Could you check a few things on this model? Use its own coordinates, in mm. Face numbers are marked on the shaded views. A direction names the side the tool comes from. Round coordinates to 2 decimals unless told otherwise and drop trailing zeros. Write each loop counter-clockwise with the first axis right and the second up, starting at its lowest first coordinate (ties: lowest second). Pieces come first, ordered by that corner, then holes. Notation, with made-up numbers: (22, 62.25) -> (35, 62.25) arc R17 cw to (35, 75.25) -> close; hole circle Ø3 at (-36, 65). An arc over 180 degrees is marked (long way). Answer as CSV lines item,"result". Start each with the question number.
Q1. Imagine slicing it at A-A on y = 5. Please give me the cut outline in (x, z).
Q2. Imagine slicing it at C-C on y = -3.5. Please give me the cut outline in (x, z) (3 decimals), and give its area (3 significant figures).
Q3. Will these pins go through, and if not, where does the flat tip stop? pin 1 Ø12 at (y, z) = (9, 8) entering from +X; pin 2 Ø4 at (y, z) = (42.5, 3) entering from +X; pin 3 Ø1.5 at (x, z) = (4, 13.5) entering from -Y; pin 4 Ø1.5 at (x, y) = (2.5, 5) entering from -Z.
Q4. If I drill on line 1 (Y direction, x = 11.7, z = 2.5) (3 decimals); line 2 (Z direction, x = 7.25, y = 1); line 3 (X direction, y = 34, z = -0.25), over which ranges is the centre line in solid material (lowest first)? Write a range as [from, to].
Q5. If we mould it in two halves opening along Z, with no side actions, what happens to the marked faces 6, 7, 8 and 9? For each: pulls with the +Z half, pulls with the -Z half, needs draft (parallel to the pull), parting line crosses it, or undercut.
Q6. Imagine slicing it at B-B on z = 7.5. Please give me the cut outline in (x, y).
Q7. Imagine slicing it at D-D on x = 14.25. Please give me the cut outline in (y, z).
Q8. For the marked faces 1, 2, 3, 4 and 5, which set-ups out of +Z, -Z, +X, -X, +Y, -Y let a thin tool reach every point of the face, with its end or its side?
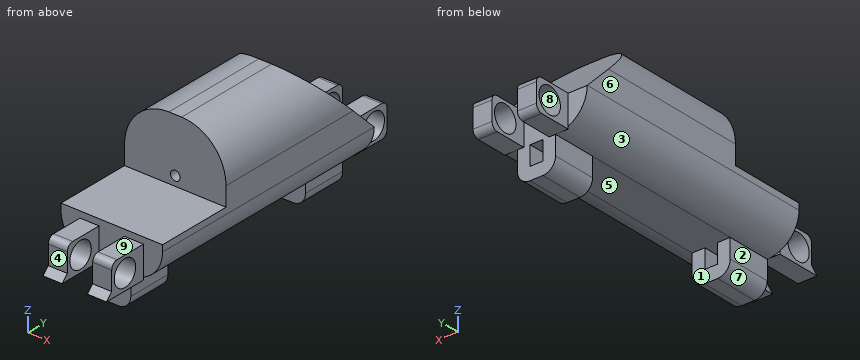
Autodesk Inventor part; units mm, degrees
ref_plane "YZ Plane" through (0, 0, 0) normal (1, 0, 0) x (0, 1, 0)
ref_plane "XZ Plane" through (0, 0, 0) normal (0, 1, 0) x (-1, 0, 0)
ref_plane "XY Plane" through (0, 0, 0) normal (0, 0, 1) x (1, 0, 0)
sketch "Sketch2" plane through (0, 0, 0) normal (0, 0, 1) x (1, 0, 0)
  line L0 (0, 0) -> (16, 0)
  line L1 (16, 0) -> (16, 40)
  line L2 (16, 40) -> (0, 40)
  line L3 (0, 40) -> (0, 0)
  dimension "d0" = 16
  dimension "d1" = 40
extrude "Extrusion1" add sketch "Sketch2" along normal blind 16
fillet "Fillet1" radius 7 2 edges at (16, 20, 16) (0, 20, 16)
fillet "Fillet2" radius 5 2 edges at (16, 20, 0) (0, 20, 0)
sketch "Sketch3" plane through (16, 0, 9) normal (1, 0, 0) x (0, 0, -1)
  line L0 (4, 0) -> (4, 40)
  line L1 (4, 40) -> (-7, 29)
  line L2 (-7, 0) -> (-7, 40)
  line L3 (4, 40) -> (19.5563, 40) construction
  line L4 (-7, 29) -> (-7, 40)
  line L5 (-7, 40) -> (4, 40)
  line L6 (1, 0) -> (12.3137, 0) construction
  line L7 (-7, 8) -> (-7, 0)
  line L8 (1, 0) -> (19.9296, 0) construction
  line L9 (-7, 17.1561) -> (-7, 8)
  point P0 (9, 0)
  dimension "d6" = 135
extrude "Extrusion2" cut sketch "Sketch3" against normal through all
sketch "Sketch4" plane through (5, 40, 0) normal (0, 1, 0) x (1, 0, 0)
  line L0 (1, -4.25) -> (5, -0.75) construction
  line L1 (-5, -5) -> (11, -5)
  line L2 (1, -5) -> (-2, -5)
  line L3 (-2, -5) -> (-2, 0)
  line L4 (-2, 0) -> (1, 0)
  line L5 (1, 0) -> (1, -5)
  line L6 (5, 0) -> (8, 0)
  line L7 (8, 0) -> (8, -5)
  line L8 (8, -5) -> (5, -5)
  line L9 (5, -5) -> (5, 0)
  point P0 (-5, 0)
  point P1 (-1.888, -0.75)
  point P2 (-1.888, -4.25)
  dimension "d58" = 3
  dimension "d79" = 4
extrude "Extrusion3" add sketch "Sketch4" along normal blind 6
sketch "Sketch6" plane through (5, 0, 0) normal (0, -1, 0) x (1, 0, 0)
  line L0 (5, 0) -> (1, 0)
  line L1 (8, 0.4174) -> (8, 5)
  line L2 (5, 0) -> (8, 0)
  line L3 (8, 0) -> (8, 5)
  line L4 (8, 5) -> (5, 5)
  line L5 (5, 5) -> (5, 0)
  line L6 (-2, 0) -> (-2, 0.4174)
  line L7 (-2, 5) -> (1, 5)
  line L8 (-2, 0) -> (1, 0)
  line L9 (1, 0) -> (1, 5)
  line L10 (1, 5) -> (-2, 5)
  line L11 (-2, 5) -> (-2, 0)
  point P0 (-5, 0)
  point P1 (-1.888, 0.75)
  point P2 (1, 0.75)
  point P3 (1, 4.25)
extrude "Extrusion5" add sketch "Sketch6" along normal blind 6
sketch "Sketch11" plane through (0, 0, 5) normal (-1, 0, 0) x (0, 0, 1)
  line L0 (0, 40) -> (0, 0)
  line L1 (11, 0) -> (11, 29)
  line L2 (0, 0) -> (11, 0)
  line L3 (11, 0) -> (11, 12)
  line L4 (11, 12) -> (0, 12)
  line L5 (0, 12) -> (0, 0)
  point P0 (-5, 0)
  dimension "d36" = 12
extrude "Extrusion9" cut sketch "Sketch11" against normal through all
sketch "Sketch12" plane through (0, 0, 0) normal (0, 0, -1) x (-1, 0, 0)
  line L0 (-10, 40) -> (-12.888, 40)
  line L1 (-11, 40) -> (-9, 40)
  line L2 (-9, 40) -> (-9, 33)
  line L3 (-9, 33) -> (-11, 33)
  line L4 (-11, 33) -> (-11, 40)
  line L5 (-5, 40) -> (-5, 0)
  line L6 (-5, 40) -> (-7, 40)
  line L7 (-7, 40) -> (-7, 33)
  line L8 (-7, 33) -> (-5, 33)
  line L9 (-5, 33) -> (-5, 40)
  line L10 (-12.888, 0) -> (-10, 0)
  line L11 (-11, 0) -> (-9, 0)
  line L12 (-9, 0) -> (-9, 7)
  line L13 (-9, 7) -> (-11, 7)
  line L14 (-11, 7) -> (-11, 0)
  line L15 (-5, 0) -> (-7, 0)
  line L16 (-7, 0) -> (-7, 7)
  line L17 (-7, 7) -> (-5, 7)
  line L18 (-5, 7) -> (-5, 0)
  point P0 (0, 0)
  point P1 (-5, 0)
  dimension "d39" = 2
  dimension "d40" = 7
  dimension "d41" = 2
  dimension "d42" = 7
  dimension "d43" = 2
  dimension "d44" = 7
  dimension "d45" = 2
  dimension "d46" = 7
extrude "Extrusion10" add sketch "Sketch12" along normal blind 3
sketch "Sketch13" plane through (0, 0, -3) normal (0, 0, -1) x (-1, 0, 0)
  line L0 (-16, 40) -> (-13, 40)
  line L1 (-11, 40) -> (-10, 40)
  line L2 (-5, 40) -> (-5, 33)
  line L3 (-11, 40) -> (-5, 40)
  line L4 (-5, 40) -> (-5, 33)
  line L5 (-5, 33) -> (-11, 33)
  line L6 (-11, 33) -> (-11, 40)
  line L7 (-11, 7) -> (-11, 33)
  line L8 (-3, 0) -> (-5, 0)
  line L9 (-11, 7) -> (-5, 7)
  line L10 (-5, 7) -> (-5, 0)
  line L11 (-5, 0) -> (-11, 0)
  line L12 (-11, 0) -> (-11, 7)
  point P0 (0, 0)
extrude "Extrusion11" add sketch "Sketch13" along normal blind 2
sketch "Sketch14" plane through (0, 12, 5) normal (0, -1, 0) x (1, 0, 0)
  circle A0 centre (8, 2.5) radius 0.75
  line L0 (16, 0) -> (0, 0)
  line L1 (16, 4) -> (16, 0)
  point P0 (0, -5)
  point P1 (16, 2)
  dimension "d52" = 1.5
  dimension "d55" = 2.5
  dimension "d56" = 8
extrude "Extrusion12" cut sketch "Sketch14" against normal through all
fillet "Fillet5" radius 2 4 edges at (11, 3.5, -5) (5, 3.5, -5) (11, 36.5, -5) (5, 36.5, -5)
sketch "Sketch15" plane through (13, 40, 0.4174) normal (1, 0, 0) x (0, 0, -1)
  circle A0 centre (-2.0826, 3.5) radius 2.025
  line L0 (0.4174, 0) -> (0.4174, 6)
  line L1 (-4.5826, 6) -> (0.4174, 6)
  point P0 (0.4174, -40)
  point P1 (0.4174, 3)
  dimension "d60" = 4.05
  dimension "d61" = 2.5
  dimension "d62" = 2.5
extrude "Extrusion13" cut sketch "Sketch15" against normal through all
fillet "Fillet6" radius 1 4 edges at (11.5, 46, 0) (11.5, 46, 5) (4.5, 46, 0) (4.5, 46, 5)
sketch "Sketch16" plane through (13, 0, 0.4174) normal (1, 0, 0) x (0, 0, -1)
  circle A0 centre (-2.0826, -3.5) radius 2.025
  line L0 (0.4174, 0) -> (0.4174, -6)
  line L1 (0.4174, -6) -> (-4.5826, -6)
  dimension "d66" = 4.05
  dimension "d67" = 2.5
  dimension "d68" = 2.5
extrude "Extrusion14" cut sketch "Sketch16" against normal through all
fillet "Fillet7" radius 1 2 edges at (4.5, -6, 5) (11.5, -6, 5)
sketch "Sketch17" plane through (5, -6, 0) normal (0, -1, 0) x (1, 0, 0)
  line L0 (8, 0) -> (8, 0.4174)
  line L1 (5, 0) -> (5, 5)
  line L2 (8, 0) -> (5, 0)
  line L3 (5, 0) -> (5, 1)
  line L4 (5, 1) -> (8, 1)
  line L5 (8, 1) -> (8, 0)
  line L6 (-2, 0) -> (1, 0)
  line L7 (-2, 0) -> (1, 0)
  line L8 (1, 0) -> (1, 1)
  line L9 (1, 1) -> (-2, 1)
  line L10 (-2, 1) -> (-2, 0)
  point P0 (-5, 0)
  dimension "d72" = 1
extrude "Extrusion15" add sketch "Sketch17" along normal blind 1
sketch "Sketch18" plane through (13, 0, 0.4174) normal (1, 0, 0) x (0, 0, -1)
  line L0 (-3.5826, -6) -> (-0.5826, -6)
  line L1 (0.4174, 0) -> (0.4174, -7)
  line L2 (-0.5826, -6) -> (0.4174, -7)
  line L3 (0.4174, -7) -> (-0.5826, -7)
  line L4 (-0.5826, -7) -> (-0.5826, -6)
extrude "Extrusion16" cut sketch "Sketch18" against normal through all
sketch "Sketch19" plane through (6, 0, 5) normal (0, 0, 1) x (-1, 0, 0)
  line L0 (-10, -12) -> (-10, -36)
  line L1 (-3, 0) -> (6, 0)
  line L2 (-10, -12) -> (6, -12)
  line L3 (6, -12) -> (6, 0)
  line L4 (6, 0) -> (-10, 0)
  line L5 (-10, 0) -> (-10, -12)
extrude "Extrusion17" add sketch "Sketch19" along normal blind 1
properties part number "FingerBase"
Checks:
1,outline,"(0, 5) arc R5 ccw to (5, 0) -> (5, -3) arc R2 ccw to (7, -5) -> (9, -5) arc R2 ccw to (11, -3) -> (11, 0) arc R5 ccw to (16, 5) -> (16, 6) -> (0, 6) -> close; hole (7, -3) -> (9, -3) -> (9, 0) -> (7, 0) -> close"
2,outline,"(3, 0) -> (6, 0) -> (6, 0.475) -> (3, 0.475) -> close; (3, 4.525) -> (6, 4.525) -> (6, 5) -> (3, 5) -> close; (10, 0) -> (13, 0) -> (13, 0.475) -> (10, 0.475) -> close; (10, 4.525) -> (13, 4.525) -> (13, 5) -> (10, 5) -> close"
2,area,"5.70 mm^2"
3,pin 1,"x = 16"
3,pin 2,"x = 13"
3,pin 3,"y = 12"
3,pin 4,"z = 0.32"
4,line 1,"[-6, -5.525], [-1.475, 41.475], [45.525, 46]"
4,line 2,"[-5, -3], [0, 6]"
4,line 3,"[5, 7], [9, 11]"
5,face 6,"needs draft"
5,face 7,"pulls with the -Z half"
5,face 8,"undercut"
5,face 9,"pulls with the +Z half"
6,outline,"(0, 12) -> (7.25, 12) -> (7.25, 37.5) -> (0, 37.5) -> close; (8.75, 12) -> (16, 12) -> (16, 37.5) -> (8.75, 37.5) -> close"
7,outline,"(0, 1.2) -> (40, 1.2) -> (40, 5) -> (31.37, 13.63) -> (12, 13.63) -> (12, 6) -> (0, 6) -> close"
8,face 1,"-Z, +X, -X"
8,face 2,"-Z, -X, +Y, -Y"
8,face 3,"-Z, -X"
8,face 4,"+Z, +X, -X, -Y"
8,face 5,"none"
